Geometry check sheet. Reference: the model listing, model coordinates, mm. A direction names the side the tool comes from. Round coordinates to 2 decimals unless told otherwise and drop trailing zeros. Write each loop counter-clockwise with the first axis right and the second up, starting at its lowest first coordinate (ties: lowest second). Pieces come first, ordered by that corner, then holes.
from build123d import *

# Parameters (mm, degrees)
SKETCH1_R           = 10.5
BOSS_EXTRUDE1_DEPTH = 5
FILLET1_R           = 15
SKETCH2_R           = 1.5
CUT_EXTRUDE1_DEPTH  = 5
SKETCH4_R           = 2.1
CUT_EXTRUDE3_DEPTH  = 10
CUT_EXTRUDE4_DEPTH  = 10


with BuildPart() as part:
    # Sketch1 → Boss-Extrude1 (new body)
    with BuildSketch(Plane.XY):
        with BuildLine():
            Line((94.301272012, 107.23010703), (12.917479745, 107.23010703))
            Line((12.917479745, 107.23010703), (50.196394157, 144.509021441))
            Line((50.196394157, 144.509021441), (33.09538699, 191.493652481))
            Line((33.09538699, 191.493652481), (-89.064653712, 147.031033848))
            Line((-89.064653712, 147.031033848), (-108.84470723, 73.210869143))
            Line((-108.84470723, 73.210869143), (-93.84470723, 47.23010703))
            Line((-93.84470723, 47.23010703), (94.301272012, 47.23010703))
            ThreePointArc((94.301272012, 47.23010703), (124.301272012, 77.23010703), (94.301272012, 107.23010703))
        make_face()
        with Locations((-17.698727988, 77.23010703)):
            Circle(SKETCH1_R, mode=Mode.SUBTRACT)
        with Locations((94.301272012, 77.23010703)):
            Circle(SKETCH1_R, mode=Mode.SUBTRACT)
    extrude(amount=BOSS_EXTRUDE1_DEPTH)

    # Fillet1
    fillet1_edges = [part.edges().sort_by_distance(p)[0] for p in [
        (12.917479745, 107.23010703, 2.5),
    ]]
    fillet(fillet1_edges, radius=FILLET1_R)

    # Sketch2 → Cut-Extrude1 (cut)
    with BuildSketch(Plane.XY.offset(5)):
        with Locations((9.098668989, 155.090939324)):
            Circle(SKETCH2_R)
        Polygon((35.831548137, 183.976111514), (10.37693066, 166.197966248), (17.217333526, 147.404113833), (47.46023301, 152.026562408), align=None)
    extrude(amount=-CUT_EXTRUDE1_DEPTH, mode=Mode.SUBTRACT)

    # Sketch4 → Cut-Extrude3 (cut)
    with BuildSketch(Plane.XY.offset(5)):
        with Locations((-83.461936193, 137.031033848)):
            Circle(SKETCH4_R)
        with Locations((-90.672471028, 110.120951496)):
            Circle(SKETCH4_R)
        with Locations((-97.883005862, 83.210869143)):
            Circle(SKETCH4_R)
    extrude(amount=-CUT_EXTRUDE3_DEPTH, mode=Mode.SUBTRACT)

    # Sketch5 → Cut-Extrude4 (cut)
    with BuildSketch(Plane.XY.offset(5)):
        with BuildLine():
            Line((-48.918590023, 116.132580639), (-85.191500994, 98.984877604))
            ThreePointArc((-85.191500994, 98.984877604), (-85.920322831, 98.239804651), (-85.987744542, 97.199723264))
            Line((-85.987744542, 97.199723264), (-83.678802495, 89.464767405))
            ThreePointArc((-83.678802495, 89.464767405), (-82.922106683, 88.557131084), (-81.742997435, 88.479069431))
            Line((-81.742997435, 88.479069431), (-47.779028512, 100.446008168))
            ThreePointArc((-47.779028512, 100.446008168), (-47.053226731, 100.994074602), (-46.777505051, 101.860759433))
            Line((-46.777505051, 101.860759433), (-46.777505051, 114.776479588))
            ThreePointArc((-46.777505051, 114.776479588), (-47.474892896, 116.043686646), (-48.918590023, 116.132580639))
        make_face()
        with BuildLine():
            Line((-40.354065156, 117.285126681), (-40.354065156, 103.938271148))
            ThreePointArc((-40.354065156, 103.938271148), (-40.239884455, 103.364246), (-39.914725328, 102.877610977))
            Line((-39.914725328, 102.877610977), (-35.506024812, 98.468910461))
            ThreePointArc((-35.506024812, 98.468910461), (-35.019389788, 98.143751334), (-34.44536464, 98.029570632))
            Line((-34.44536464, 98.029570632), (2.900545466, 98.029570632))
            ThreePointArc((2.900545466, 98.029570632), (3.153402247, 98.05103641), (3.399022006, 98.114819368))
            Line((3.399022006, 98.114819368), (26.404973303, 106.220786324))
            ThreePointArc((26.404973303, 106.220786324), (27.403506638, 107.540872748), (26.579216219, 108.976227162))
            Line((26.579216219, 108.976227162), (24.498135227, 110.020453731))
            ThreePointArc((24.498135227, 110.020453731), (24.269772253, 110.112435549), (24.029439243, 110.16582419))
            Line((24.029439243, 110.16582419), (-38.650041684, 118.771186715))
            ThreePointArc((-38.650041684, 118.771186715), (-39.839956832, 118.415621088), (-40.354065156, 117.285126681))
        make_face()
        with BuildLine():
            Line((-74.392110194, 114.92256466), (-80.203002255, 120.733456721))
            ThreePointArc((-80.203002255, 120.733456721), (-80.642342083, 121.794116893), (-80.203002255, 122.854777065))
            Line((-80.203002255, 122.854777065), (-68.473782604, 134.583996716))
            ThreePointArc((-68.473782604, 134.583996716), (-68.141065775, 134.834861797), (-67.752173145, 134.98451573))
            Line((-67.752173145, 134.98451573), (-7.313265805, 149.008705779))
            ThreePointArc((-7.313265805, 149.008705779), (-6.796836559, 149.037001955), (-6.301495636, 148.888216166))
            Line((-6.301495636, 148.888216166), (13.97461757, 138.714245904))
            ThreePointArc((13.97461757, 138.714245904), (14.427382099, 138.365164015), (14.716649378, 137.87203287))
            Line((14.716649378, 137.87203287), (20.14067974, 122.477820308))
            ThreePointArc((20.14067974, 122.477820308), (20.07878483, 121.331439698), (19.224405015, 120.564592504))
            Line((19.224405015, 120.564592504), (16.778026718, 119.70263025))
            ThreePointArc((16.778026718, 119.70263025), (16.431032479, 119.625050079), (16.075526706, 119.631321481))
            Line((16.075526706, 119.631321481), (-44.068033081, 127.888523484))
            ThreePointArc((-44.068033081, 127.888523484), (-44.500043445, 127.885036207), (-44.913141524, 127.758564501))
            Line((-44.913141524, 127.758564501), (-72.690365051, 114.627123781))
            ThreePointArc((-72.690365051, 114.627123781), (-73.588027819, 114.505331793), (-74.392110194, 114.92256466))
        make_face()
        with BuildLine():
            Line((-85.765173696, 78.039759187), (-78.678992966, 54.30105374))
            ThreePointArc((-78.678992966, 54.30105374), (-78.137884303, 53.527281204), (-77.241664446, 53.23010703))
            Line((-77.241664446, 53.23010703), (-37.000229644, 53.23010703))
            ThreePointArc((-37.000229644, 53.23010703), (-35.797403818, 53.833887172), (-35.562901123, 55.159160319))
            Line((-35.562901123, 55.159160319), (-46.478753465, 91.727265664))
            ThreePointArc((-46.478753465, 91.727265664), (-47.235449276, 92.634901985), (-48.414558525, 92.712963639))
            Line((-48.414558525, 92.712963639), (-84.826321716, 79.88356374))
            ThreePointArc((-84.826321716, 79.88356374), (-85.664534787, 79.149445185), (-85.765173696, 78.039759187))
        make_face()
        with BuildLine():
            Line((-71.137681218, 144.818765729), (-68.657481405, 142.605973483))
            ThreePointArc((-68.657481405, 142.605973483), (-68.030328991, 142.271974344), (-67.319826927, 142.264075548))
            Line((-67.319826927, 142.264075548), (-6.252231197, 156.434145889))
            ThreePointArc((-6.252231197, 156.434145889), (-5.572632004, 156.794256335), (-5.160840216, 157.443842448))
            Line((-5.160840216, 157.443842448), (-2.289133326, 166.54233045))
            ThreePointArc((-2.289133326, 166.54233045), (-1.989907511, 167.075911596), (-1.502525339, 167.445646022))
            Line((-1.502525339, 167.445646022), (8.200620604, 172.056821639))
            ThreePointArc((8.200620604, 172.056821639), (8.310747045, 172.114876187), (8.415680154, 172.181862799))
            Line((8.415680154, 172.181862799), (10.823804629, 173.863757519))
            ThreePointArc((10.823804629, 173.863757519), (11.295841918, 175.785341043), (9.451881159, 176.503053489))
            Line((9.451881159, 176.503053489), (-70.652107667, 147.347585911))
            ThreePointArc((-70.652107667, 147.347585911), (-71.612166791, 146.220903478), (-71.137681218, 144.818765729))
        make_face()
        with BuildLine():
            Line((19.452688101, 140.902959313), (26.597478805, 119.959650962))
            ThreePointArc((26.597478805, 119.959650962), (26.886716152, 119.457994505), (27.344420536, 119.103277518))
            Line((27.344420536, 119.103277518), (29.242952451, 118.150648824))
            ThreePointArc((29.242952451, 118.150648824), (30.907279592, 118.365854413), (31.330423172, 119.989814938))
            Line((31.330423172, 119.989814938), (28.480406053, 128.078591439))
            ThreePointArc((28.480406053, 128.078591439), (28.42405424, 128.870079474), (28.779368612, 129.579572626))
            Line((28.779368612, 129.579572626), (36.555739431, 138.234681359))
            ThreePointArc((36.555739431, 138.234681359), (36.911053804, 138.944174511), (36.854701991, 139.735662546))
            Line((36.854701991, 139.735662546), (35.391422248, 143.888670161))
            ThreePointArc((35.391422248, 143.888670161), (34.74811051, 144.676615426), (33.750036797, 144.872973762))
            Line((33.750036797, 144.872973762), (20.645715101, 142.870055583))
            ThreePointArc((20.645715101, 142.870055583), (19.589797516, 142.165132082), (19.452688101, 140.902959313))
        make_face()
        with BuildLine():
            Line((29.815786136, 90.775099636), (21.291462651, 87.771620945))
            ThreePointArc((21.291462651, 87.771620945), (21.219404291, 87.744129544), (21.148854219, 87.712970731))
            Line((21.148854219, 87.712970731), (6.195871701, 80.644078358))
            ThreePointArc((6.195871701, 80.644078358), (5.569749615, 80.090589463), (5.336956673, 79.287977308))
            Line((5.336956673, 79.287977308), (5.336956673, 69.717357349))
            ThreePointArc((5.336956673, 69.717357349), (5.615715461, 68.846398164), (6.348383209, 68.299155681))
            Line((6.348383209, 68.299155681), (28.762867567, 60.577318579))
            ThreePointArc((28.762867567, 60.577318579), (29.627673329, 60.543470228), (30.367229735, 60.9930156))
            Line((30.367229735, 60.9930156), (41.497463613, 73.380977374))
            ThreePointArc((41.497463613, 73.380977374), (41.852777986, 74.090470526), (41.796426172, 74.88195856))
            Line((41.796426172, 74.88195856), (40.058915507, 79.813274708))
            ThreePointArc((40.058915507, 79.813274708), (39.949210994, 80.054293252), (39.798832512, 80.272264193))
            Line((39.798832512, 80.272264193), (31.468930944, 90.317814397))
            ThreePointArc((31.468930944, 90.317814397), (30.714168094, 90.806057767), (29.815786136, 90.775099636))
        make_face()
        with BuildLine():
            Line((42.24427744, 91.095227742), (46.46113264, 82.175221783))
            ThreePointArc((46.46113264, 82.175221783), (47.311640972, 81.404082975), (48.458318662, 81.460205704))
            Line((48.458318662, 81.460205704), (57.693632468, 85.826119946))
            ThreePointArc((57.693632468, 85.826119946), (57.85814362, 85.916908827), (58.010013522, 86.027552727))
            Line((58.010013522, 86.027552727), (63.502078057, 90.581644445))
            ThreePointArc((63.502078057, 90.581644445), (63.955640452, 92.245231959), (62.544612032, 93.236312714))
            Line((62.544612032, 93.236312714), (43.60037849, 93.236312714))
            ThreePointArc((43.60037849, 93.236312714), (42.333171432, 92.538924869), (42.24427744, 91.095227742))
        make_face()
        with BuildLine():
            Line((51.268567993, 69.307256916), (41.511994194, 61.21697836))
            ThreePointArc((41.511994194, 61.21697836), (41.058431799, 59.553390846), (42.469460219, 58.562310092))
            Line((42.469460219, 58.562310092), (61.622416924, 58.562310092))
            ThreePointArc((61.622416924, 58.562310092), (63.028666211, 59.540330264), (62.601128605, 61.19902617))
            Line((62.601128605, 61.19902617), (53.2047457, 69.289304726))
            ThreePointArc((53.2047457, 69.289304726), (52.239941382, 69.652524174), (51.268567993, 69.307256916))
        make_face()
        with BuildLine():
            Line((67.498580228, 69.401810839), (60.046591123, 75.731258856))
            ThreePointArc((60.046591123, 75.731258856), (59.554291768, 77.204084461), (60.630425962, 78.323686674))
            Line((60.630425962, 78.323686674), (68.082415068, 80.314857078))
            ThreePointArc((68.082415068, 80.314857078), (69.383188538, 80.055407885), (69.969630372, 78.865697215))
            Line((69.969630372, 78.865697215), (69.969630372, 70.545078794))
            ThreePointArc((69.969630372, 70.545078794), (69.099481459, 69.183723731), (67.498580228, 69.401810839))
        make_face()
    extrude(amount=-CUT_EXTRUDE4_DEPTH, mode=Mode.SUBTRACT)


solid = part.part
1. Section check A-A (z = 2.9). State how many separate pieces and enclosed holes the cut face has, plus the area to 3 significant figures.
2. Depth check by flat-ended pin: pin 1 Ø2 at (y, z) = (94, 4.5) entering from +X; pin 2 Ø1.5 at (y, z) = (151.5, 0.5) entering from +X; pin 3 Ø2.5 at (x, z) = (-57.5, 1.5) entering from +Y. Enter the tip coordinate at first touch or a pass-through.
3. Section check B-B (x = 109.5). Record the cut outline in (y, z), plus the area to 3 significant figures.
4. Scan lines: line 1 along Y through (x, z) = (7, 3.05); line 2 along X through (y, z) = (109, 2); line 3 along Y through (x, z) = (-16.5, 4.45). Record each from-to range of solid material in increasing order.
5. Release check for a two-part mould opening along Y. For faces 3 (the face through (35.692, 85.225, 2.535)), 4 (the face through (6, 88, 5)) record: +Y half, -Y half, draft (parallel to the pull), parting line (faces both ways), or undercut.
6. Access from +Z, -Z, +X, -X, +Y, -Y to the whole of each face (thin tool, end or side, straight path). Record for faces 1 (the face through (53, 93.236, 3)), 2 (the face through (44.28, 138.59, 2.46)).
Results below:
1. separate pieces: 1
1. enclosed holes: 16
1. area: 13,300 mm2
2. pin 1: stops at x = 119.82
2. pin 2: stops at x = 47.92
2. pin 3: stops at y = 158.97
3. outline: (51.37, 0) - (103.1, 0) - (103.1, 5) - (51.37, 5) - close
3. area: 259 mm2
4. line 1: y = 47.23 to 68.07, 81.02 to 99.38, 112.5 to 120.88, 142.21 to 171.49, 175.61 to 182
4. line 2: x = -99.26 to -92.45, -88.9 to -64.01, -46.78 to -40.35, 26.53 to 42.06
4. line 3: y = 47.23 to 66.8, 87.66 to 98.03, 115.73 to 124.1, 146.88 to 154.06, 167.06 to 173.44
5. face 3: undercut
5. face 4: draft
6. face 1: +Z, -Z
6. face 2: +Z, -Z, +X
